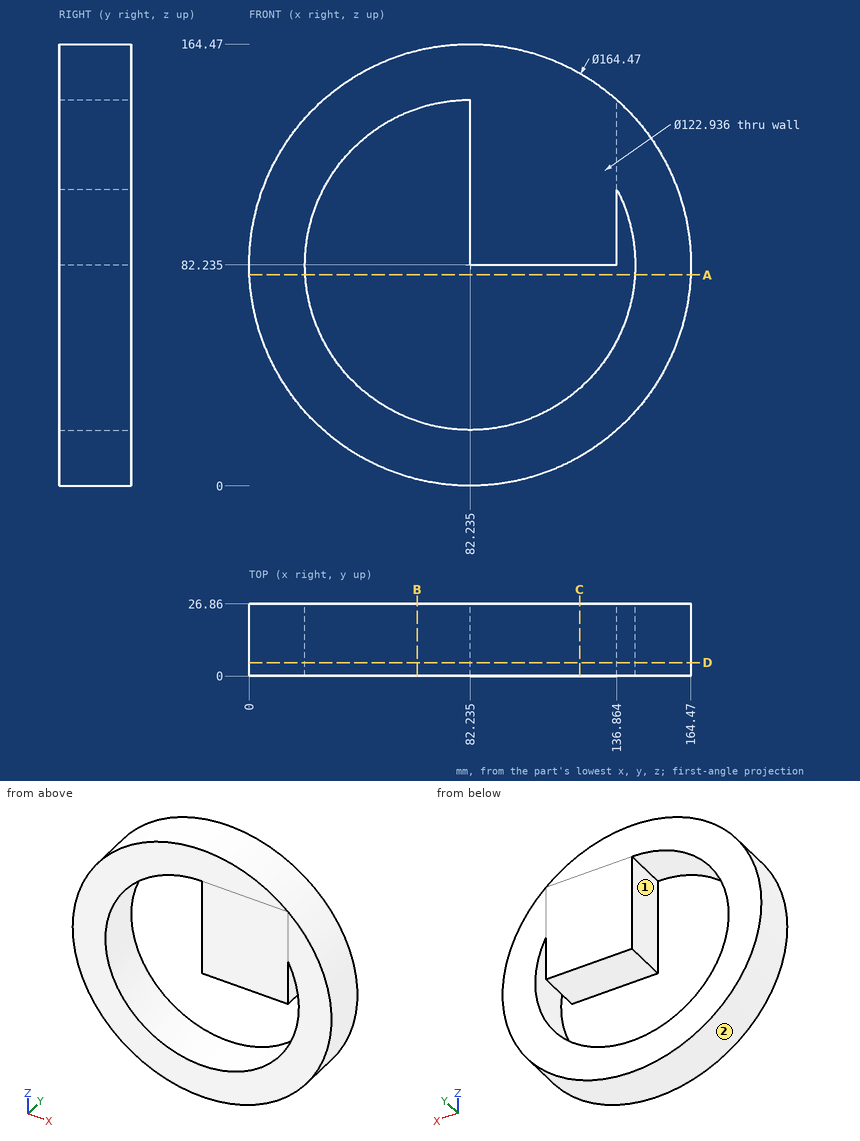
Geometry: see drawing. Coordinates: mm, zero at the bounding-box minimum. Round coordinates to 2 decimals unless told otherwise and drop trailing zeros. Loops run counter-clockwise (first coordinate to the right, second up) from the corner with the lowest first, then second, coordinate; pieces in that order, holes last. Notation, with made-up numbers: (70.5, 29) -> (116.5, 29) arc R21 ccw to (116.5, 58) -> close; hole circle Ø9 at (20.25, -39.75). An arc over 180 degrees is marked (long way). One line per question, with ' | ' between items. Start each with the question number.
1. Section B-B on x = 62.5. Output: boundary loops of the cut face in (y, z).
2. Contact query for flat-ended pins moving along their axis: pin 1 (10 mm diameter, centred on x = 37.5, y = 14, fed in from +Z); pin 2 (8 mm diameter, centred on y = 8.5, z = 102.5, fed in from -X) (1 decimal); pin 3 (1 mm diameter, centred on y = 3, z = 112.5, fed in from +X) (1 decimal). Output: stop coordinate, or through.
3. Section C-C on x = 123. Output: boundary loops of the cut face in (y, z) (1 decimal).
4. Mould query, pull axis Z, two halves, no side actions, for the marked faces 1 and 2. Classes: pulls with the +Z half, pulls with the -Z half, needs draft (parallel to the pull), parting line crosses it, or undercut.
5. Line query: line 1 along X through (y, z) = (17.5, 83.5) (1 decimal); line 2 along X through (y, z) = (1.5, 84.5) (1 decimal); line 3 along Z through (x, y) = (112, 21) (1 decimal). Output: solid intervals per line, ascending. Write a range as [from, to].
6. Section A-A on z = 78.5. Output: boundary loops of the cut face in (x, y) (1 decimal), and give its area (3 significant figures).
7. Section D-D on y = 5. Output: boundary loops of the cut face in (x, z) (1 decimal).
Returned:
1) outline: (0, 2.4) -> (26.86, 2.4) -> (26.86, 24.02) -> (0, 24.02) -> close; (0, 140.45) -> (26.86, 140.45) -> (26.86, 162.07) -> (0, 162.07) -> close
2) pin 1: stops at z = 154.23 | pin 2: stops at x = 1.6 | pin 3: stops at x = 158.9
3) outline: (0, 10.8) -> (26.9, 10.8) -> (26.9, 36.2) -> (0, 36.2) -> close; (0, 82.2) -> (26.9, 82.2) -> (26.9, 153.7) -> (0, 153.7) -> close
4) face 1: undercut | face 2: parting line crosses it
5) line 1: x = [0, 20.8], [82.2, 136.9], [143.7, 164.5] | line 2: x = [0, 20.8], [82.2, 136.9], [143.7, 164.4] | line 3: z = [5.6, 28.5], [82.2, 158.9]
6) outline: (0.1, 0) -> (20.9, 0) -> (20.9, 26.9) -> (0.1, 26.9) -> close; (143.6, 0) -> (164.4, 0) -> (164.4, 26.9) -> (143.6, 26.9) -> close | area: 1,120 mm2
7) outline: circle Ø164.5 at (82.2, 82.2); hole (82.2, 82.2) -> (82.2, 143.7) arc R61.5 ccw (long way) to (136.9, 110.4) -> (136.9, 82.2) -> close
